```python
from build123d import *

# Parameters (mm, degrees)
SKETCH1_R           = 107.5
SKETCH1_R_2         = 94.17
SKETCH1_R_3         = 2
BOSS_EXTRUDE1_DEPTH = 4
SKETCH2_R           = 3.6
CUT_EXTRUDE1_DEPTH  = 10


with BuildPart() as part:
    # Sketch1 → Boss-Extrude1 (new body)
    with BuildSketch(Plane(origin=(0, 0, 0), x_dir=(1, 0, 0), z_dir=(0, 1, 0))):
        with Locations(Location((0, 0, 0), (0, 0, 270))):
            Circle(SKETCH1_R)
        with Locations(Location((0, 0, 0), (0, 0, 270))):
            Circle(SKETCH1_R_2, mode=Mode.SUBTRACT)
        with Locations(Location((86.749764697, 50.085, 0), (0, 0, 270))):
            Circle(SKETCH1_R_3, mode=Mode.SUBTRACT)
        with Locations(Location((96.756790019, -25.925903748, 0), (0, 0, 270))):
            Circle(SKETCH1_R_3, mode=Mode.SUBTRACT)
        with Locations(Location((50.085, -86.749764697, 0), (0, 0, 270))):
            Circle(SKETCH1_R_3, mode=Mode.SUBTRACT)
        with Locations(Location((-25.925903748, -96.756790019, 0), (0, 0, 270))):
            Circle(SKETCH1_R_3, mode=Mode.SUBTRACT)
        with Locations(Location((-86.749764697, -50.085, 0), (0, 0, 270))):
            Circle(SKETCH1_R_3, mode=Mode.SUBTRACT)
        with Locations(Location((-96.756790019, 25.925903748, 0), (0, 0, 270))):
            Circle(SKETCH1_R_3, mode=Mode.SUBTRACT)
        with Locations(Location((-50.085, 86.749764697, 0), (0, 0, 270))):
            Circle(SKETCH1_R_3, mode=Mode.SUBTRACT)
        with Locations(Location((25.925903748, 96.756790019, 0), (0, 0, 270))):
            Circle(SKETCH1_R_3, mode=Mode.SUBTRACT)
    extrude(amount=BOSS_EXTRUDE1_DEPTH)

    # Sketch2 → Cut-Extrude1 (cut)
    with BuildSketch(Plane(origin=(0, 4, 0), x_dir=(1, 0, 0), z_dir=(0, 1, 0))):
        with Locations(Location((96.756790019, 25.925903748, 0), (0, 0, 270))):
            Circle(SKETCH2_R)
        with Locations(Location((86.749764697, -50.085, 0), (0, 0, 270))):
            Circle(SKETCH2_R)
        with Locations(Location((25.925903748, -96.756790019, 0), (0, 0, 270))):
            Circle(SKETCH2_R)
        with Locations(Location((-50.085, -86.749764697, 0), (0, 0, 270))):
            Circle(SKETCH2_R)
        with Locations(Location((-96.756790019, -25.925903748, 0), (0, 0, 270))):
            Circle(SKETCH2_R)
        with Locations(Location((-86.749764697, 50.085, 0), (0, 0, 270))):
            Circle(SKETCH2_R)
        with Locations(Location((-25.925903748, 96.756790019, 0), (0, 0, 270))):
            Circle(SKETCH2_R)
        with Locations(Location((50.085, 86.749764697, 0), (0, 0, 270))):
            Circle(SKETCH2_R)
    extrude(amount=-CUT_EXTRUDE1_DEPTH, mode=Mode.SUBTRACT)


solid = part.part
```
Here's how the part is built. I have some questions about the finished solid (model axes, mm). Coordinates: 2 decimals unless noted, no trailing zeros. Order: outer loops, then holes, each group sorted by start corner. A loop starts at its lowest first (then second) coordinate and runs counter-clockwise, first axis right, second up.
Item 1: I need wall thicknesses on probe 1 along Z at (x, y) = (84, 2.6); probe 2 along Z at (x, y) = (-98, 2.4); probe 3 along X at (y, z) = (1.4, -53). Which ranges of each line are inside material? Lowest first, please.
Response values:
probe 1: z = -67.08 to -42.57, 42.57 to 47.76, 52.41 to 67.08
probe 2: z = -44.18 to -27.49, -24.36 to 22.55, 29.3 to 44.18
probe 3: x = -93.53 to -88.86, -84.64 to -77.84, 77.84 to 93.53
Item 2: I'm going to push flat-ended pins straight in: pin 1 Ø1 at (y, z) = (3.5, -45.5) entering from -X; pin 2 Ø3 at (x, z) = (86.75, -50.08) entering from -Y; pin 3 Ø1 at (y, z) = (3.5, 20) entering from -X. Where does each tip first touch, or does it pass through?
Response values:
pin 1: stops at x = -97.63
pin 2: passes through
pin 3: stops at x = -105.72
Item 3: If we section it at B-B, the plane z = 0: List the corners of the cut face in (x, y) for me.
Response values:
outline: (-107.5, 0) - (-94.17, 0) - (-94.17, 4) - (-107.5, 4) - close; (94.17, 0) - (107.5, 0) - (107.5, 4) - (94.17, 4) - close
Item 4: Thinking about a two-plate mould opening in X: for faces 1 (the face through (-95, 4, -1)), 2 (the face through (-104.944, 1.972, -23.304)), 3 (the face through (26.08, 2.03, 93.16)), which applies, pulls with the +X half, pulls with the -X half, needs draft (parallel to the pull), parting line crosses it, or undercut?
Response values:
face 1: needs draft
face 2: parting line crosses it
face 3: undercut
Item 5: If we section it at C-C, the plane y = 3.3: Give the number of separate pieces and of enclosed holes in the cut face, then the cut area to 3 significant figures.
Response values:
separate pieces: 1
enclosed holes: 17
area: 8,020 mm2
Item 6: If we section it at A-A, the plane x = 0: List the corners of the cut face in (y, z) for me, then the cut area to 3 significant figures.
Response values:
outline: (0, -107.5) - (4, -107.5) - (4, -94.17) - (0, -94.17) - close; (0, 94.17) - (4, 94.17) - (4, 107.5) - (0, 107.5) - close
area: 107 mm2
